Autodesk Inventor part; units mm, degrees
ref_plane "YZ Plane" through (0, 0, 0) normal (1, 0, 0) x (0, 1, 0)
ref_plane "XZ Plane" through (0, 0, 0) normal (0, 1, 0) x (-1, 0, 0)
ref_plane "XY Plane" through (0, 0, 0) normal (0, 0, 1) x (1, 0, 0)
sketch "Sketch1" plane through (0, 0, 0) normal (1, 0, 0) x (0, 1, 0)
  line L0 (136.2492, 38.7083) -> (-163.7508, 38.7083)
  line L1 (-163.7508, -36.2917) -> (136.2492, -36.2917)
  line L2 (-160.7508, 13.7083) -> (-160.7508, -11.2917)
  line L3 (-160.7508, -11.2917) -> (-163.7508, -11.2917)
  line L4 (-160.7508, 13.7083) -> (-163.7508, 13.7083)
  line L5 (-163.7508, 13.7083) -> (-163.7508, 38.7083)
  line L6 (-163.7508, -11.2917) -> (-163.7508, -36.2917)
  line L7 (136.2492, 38.7083) -> (136.2492, 13.7083)
  line L8 (136.2492, -36.2917) -> (136.2492, -11.2917)
  line L9 (136.2492, 13.7083) -> (133.2492, 13.7083)
  line L10 (133.2492, 13.7083) -> (133.2492, -11.2917)
  line L11 (136.2492, -11.2917) -> (133.2492, -11.2917)
  point P0 (0, 0)
  dimension "d1" = 300
extrude "Extrusion1" add sketch "Sketch1" along normal blind 3
sketch "Sketch2" plane through (3, 0, 0) normal (1, 0, 0) x (0, 0, -1)
  line L0 (-13.7083, -163.7508) -> (-13.7083, -160.7508)
  line L1 (-13.7083, -160.7508) -> (11.2917, -160.7508)
  line L2 (-13.7083, -60.7508) -> (11.2917, -60.7508)
  line L3 (11.2917, -60.7508) -> (11.2917, -63.7508)
  line L4 (11.2917, -63.7508) -> (-13.7083, -63.7508)
  line L5 (-13.7083, -63.7508) -> (-13.7083, -60.7508)
  line L6 (36.2917, -163.7508) -> (36.2917, 136.2492)
  line L7 (-13.7083, 36.2492) -> (11.2917, 36.2492)
  line L8 (11.2917, 36.2492) -> (11.2917, 39.2492)
  line L9 (11.2917, 39.2492) -> (-13.7083, 39.2492)
  line L10 (-13.7083, 39.2492) -> (-13.7083, 36.2492)
  point P0 (0, 0)
extrude "Extrusion2" cut sketch "Sketch2" against normal blind 3
sketch "Sketch3" plane through (3, 0, 0) normal (1, 0, 0) x (0, 0, -1)
  line L0 (-13.7083, -160.7508) -> (11.2917, -160.7508)
  circle A0 centre (-16.7083, -154.7508) radius 1.5
  circle A1 centre (14.2917, -154.7508) radius 1.5
  circle A2 centre (14.2917, -123.7508) radius 1.5
  circle A3 centre (-16.7083, -123.7508) radius 1.5
  circle A4 centre (-1.2083, -139.2508) radius 12
  point P0 (0, 0)
  dimension "d29" = 3
  dimension "d30" = 3
  dimension "d31" = 3
  dimension "d32" = 3
  dimension "d33" = 24
extrude "Extrusion3" cut sketch "Sketch3" against normal blind 3
sketch "Sketch4" plane through (3, 0, 0) normal (1, 0, 0) x (0, 0, -1)
  line L0 (-13.7083, -160.7508) -> (11.2917, -160.7508)
  line L1 (36.2917, -163.7508) -> (36.2917, 136.2492)
  line L2 (31.2917, -155.7508) -> (28.2917, -155.7508)
  line L3 (28.2917, -155.7508) -> (28.2917, -145.7508)
  line L4 (28.2917, -145.7508) -> (31.2917, -145.7508)
  line L5 (31.2917, -145.7508) -> (31.2917, -155.7508)
  line L6 (-38.7083, 136.2492) -> (-38.7083, -163.7508)
  line L7 (-33.7083, -155.7508) -> (-30.7083, -155.7508)
  line L8 (-30.7083, -155.7508) -> (-30.7083, -145.7508)
  line L9 (-30.7083, -145.7508) -> (-33.7083, -145.7508)
  line L10 (-33.7083, -145.7508) -> (-33.7083, -155.7508)
  line L11 (-33.7083, 128.1373) -> (-30.7083, 128.1373)
  line L12 (-30.7083, 128.1373) -> (-30.7083, 118.1373)
  line L13 (-30.7083, 118.1373) -> (-33.7083, 118.1373)
  line L14 (-33.7083, 118.1373) -> (-33.7083, 128.1373)
  line L15 (31.2917, 128.1373) -> (28.2917, 128.1373)
  line L16 (28.2917, 128.1373) -> (28.2917, 118.1373)
  line L17 (28.2917, 118.1373) -> (31.2917, 118.1373)
  line L18 (31.2917, 118.1373) -> (31.2917, 128.1373)
  point P0 (0, 0)
  dimension "d38" = 3
  dimension "d39" = 10
  dimension "d46" = 3
  dimension "d47" = 10
  dimension "d48" = 3
  dimension "d49" = 10
  dimension "d50" = 10
  dimension "d51" = 3
extrude "Extrusion4" cut sketch "Sketch4" against normal blind 30
sketch "Sketch5" plane through (3, 0, 0) normal (1, 0, 0) x (0, 0, -1)
  line L0 (-13.7083, -60.7508) -> (11.2917, -60.7508)
  line L1 (-38.7083, 136.2492) -> (-38.7083, -163.7508)
  line L2 (36.2917, -163.7508) -> (36.2917, 136.2492)
  line L3 (-28.7083, -55.7508) -> (26.2917, -55.7508)
  line L4 (26.2917, -55.7508) -> (26.2917, -43.2508)
  line L5 (26.2917, -43.2508) -> (-28.7083, -43.2508)
  line L6 (-28.7083, -43.2508) -> (-28.7083, -55.7508)
  point P0 (0, 0)
extrude "Extrusion5" cut sketch "Sketch5" against normal blind 10
sketch "Sketch6" plane through (3, 0, 0) normal (1, 0, 0) x (0, 0, -1)
  line L0 (-30.7083, 118.1373) -> (-33.7083, 118.1373)
  line L1 (-33.7083, 118.1373) -> (-30.7083, 118.1373)
  line L2 (-30.7083, 118.1373) -> (-30.7083, 103.1373)
  line L3 (-30.7083, 103.1373) -> (-33.7083, 103.1373)
  line L4 (-33.7083, 103.1373) -> (-33.7083, 118.1373)
  line L5 (28.2917, 118.1373) -> (31.2917, 118.1373)
  line L6 (28.2917, 118.1373) -> (31.2917, 118.1373)
  line L7 (31.2917, 118.1373) -> (31.2917, 103.1373)
  line L8 (31.2917, 103.1373) -> (28.2917, 103.1373)
  line L9 (28.2917, 103.1373) -> (28.2917, 118.1373)
  line L10 (-33.7083, -155.7508) -> (-33.7083, -145.7508)
  line L11 (-33.7083, -145.7508) -> (-30.7083, -145.7508)
  line L12 (-30.7083, -145.7508) -> (-30.7083, -130.7508)
  line L13 (-30.7083, -130.7508) -> (-33.7083, -130.7508)
  line L14 (-33.7083, -130.7508) -> (-33.7083, -145.7508)
  line L15 (28.2917, -155.7508) -> (28.2917, -145.7508)
  line L16 (28.2917, -145.7508) -> (31.2917, -145.7508)
  line L17 (31.2917, -145.7508) -> (31.2917, -130.7508)
  line L18 (31.2917, -130.7508) -> (28.2917, -130.7508)
  line L19 (28.2917, -130.7508) -> (28.2917, -145.7508)
  point P0 (0, 0)
  dimension "d62" = 15
  dimension "d63" = 15
extrude "Extrusion6" cut sketch "Sketch6" against normal blind 10
sketch "Sketch7" plane through (3, 0, 0) normal (1, 0, 0) x (0, 0, -1)
  point P0 (0, 0)
sketch "Sketch8" plane through (3, 0, 0) normal (1, 0, 0) x (0, 0, -1)
  circle A0 centre (-16.7083, -123.7508) radius 1.5
  circle A1 centre (14.2917, -123.7508) radius 1.5
  line L0 (-16.7083, -123.7508) -> (14.2917, -123.7508)
  circle A2 centre (14.2917, -154.7508) radius 1.5
  line L1 (14.2917, -123.7508) -> (14.2917, -154.7508)
  circle A3 centre (-16.7083, -154.7508) radius 1.5
  line L2 (14.2917, -154.7508) -> (-16.7083, -154.7508)
  line L3 (-16.7083, -154.7508) -> (-16.7083, -123.7508)
  circle A4 centre (-16.7083, -123.7508) radius 1.5
  circle A5 centre (14.2917, -123.7508) radius 1.5
  circle A6 centre (14.2917, -154.7508) radius 1.5
  circle A7 centre (-16.7083, -154.7508) radius 1.5
  circle A8 centre (-1.2083, -139.2508) radius 12
  circle A9 centre (-1.2083, -139.2508) radius 12
  point P0 (0, 0)
extrude "Extrusion7" add sketch "Sketch8" against normal blind 3 contours L0 L3 A0 | A0 L3 L0 | L0 L1 A1 | A1 L1 L0 | L3 L2 A3 | A3 L2 L3 | L1 L2 A2 | A2 L2 L1 | A8
sketch "Sketch9" plane through (3, 0, 0) normal (1, 0, 0) x (0, 0, -1)
  line L0 (11.2917, -163.7508) -> (36.2917, -163.7508)
  line L1 (-38.7083, -163.7508) -> (-13.7083, -163.7508)
  line L2 (36.2917, -163.7508) -> (36.2917, 136.2492)
  circle A0 centre (-16.7083, -153.7508) radius 2
  circle A1 centre (14.2917, -153.7508) radius 2
  circle A2 centre (14.2917, -122.7508) radius 2
  circle A3 centre (-16.7083, -122.7508) radius 2
  circle A4 centre (-1.2083, -138.2508) radius 12
  point P0 (0, 0)
  dimension "d75" = 4
  dimension "d76" = 4
  dimension "d77" = 4
  dimension "d78" = 4
  dimension "d79" = 24
extrude "Extrusion8" cut sketch "Sketch9" against normal blind 3
sketch "Sketch10" plane through (3, 0, 0) normal (1, 0, 0) x (0, 0, -1)
  circle A0 centre (-1.2083, -138.2508) radius 12
  circle A1 centre (-1.2083, -138.2508) radius 13.75
  point P0 (0, 0)
  dimension "d82" = 27.5
extrude "Extrusion9" cut sketch "Sketch10" against normal blind 10 contours A0 | A1
properties part number "MuurL"
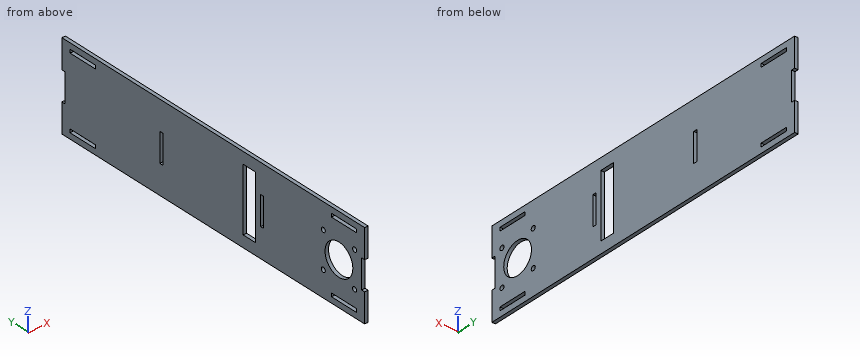
The listing builds one solid part. Answer for the finished solid, in the listing's coordinates (mm). Round coordinates to 2 decimals unless told otherwise and drop trailing zeros. Order: outer loops, then holes, each group sorted by start corner. A loop starts at its lowest first (then second) coordinate and runs counter-clockwise, first axis right, second up. Notation, with made-up numbers: (28, 1.5) - (53, 1.5) arc R28 cw to (53, 27.5) - close; hole circle Ø6 at (-21.75, 68). An arc over 180 degrees is marked (long way). Put each result on its own line as item: value. Start each with the question number.
(1) Find section B-B (z = -3). Give the vertices of the cut face in (x, y), plus the area to 3 significant figures.
(2) Find section C-C (x = 2.35). State how many separate pieces and enclosed holes the cut face has, plus the area to 3 significant figures.
(3) Given P1, Ø0.9, axis at x = 2, z = 4.5, coming from the +Y side; P2, Ø5, axis at y = -153.75, z = 16.71, coming from the +X side; P3, Ø1.5, axis at x = 1, z = -4, coming from the -Y side, each flat-ended and moving along its own axis, determine where each tip first touches the part or whether it passes through.
(4) Find section A-A (y = -53). Give the vertices of the cut face in (x, z), plus the area to 3 significant figures.
(5) Straight lines are drawn through the part: probe 1 along Z at (x, y) = (2.1, 115); probe 2 along Y at (x, z) = (2.2, 32); probe 3 along Z at (x, y) = (0.1, -139.5). For each, find the intervals that lie inside material, in ascending order. Write a range as from..to.
Reply:
1. outline: (0, -160.75) - (3, -160.75) - (3, -151.34) - (0, -151.34) - close; (0, -125.16) - (3, -125.16) - (3, -63.75) - (0, -63.75) - close; (0, -60.75) - (3, -60.75) - (3, -55.75) - (0, -55.75) - close; (0, -43.25) - (3, -43.25) - (3, 36.25) - (0, 36.25) - close; (0, 39.25) - (3, 39.25) - (3, 133.25) - (0, 133.25) - close
1. area: 748 mm^2
2. separate pieces: 1
2. enclosed holes: 12
2. area: 20,600 mm^2
3. P1: y = 133.25
3. P2: x = 3
3. P3: y = -160.75
4. outline: (0, -36.29) - (3, -36.29) - (3, -26.29) - (0, -26.29) - close; (0, 28.71) - (3, 28.71) - (3, 38.71) - (0, 38.71) - close
4. area: 60.0 mm^2
5. probe 1: -36.29..-31.29, -28.29..30.71, 33.71..38.71
5. probe 2: -163.75..-155.75, -130.75..103.14, 128.14..136.25
5. probe 3: -36.29..-31.29, -28.29..-12.48, 14.9..30.71, 33.71..38.71
